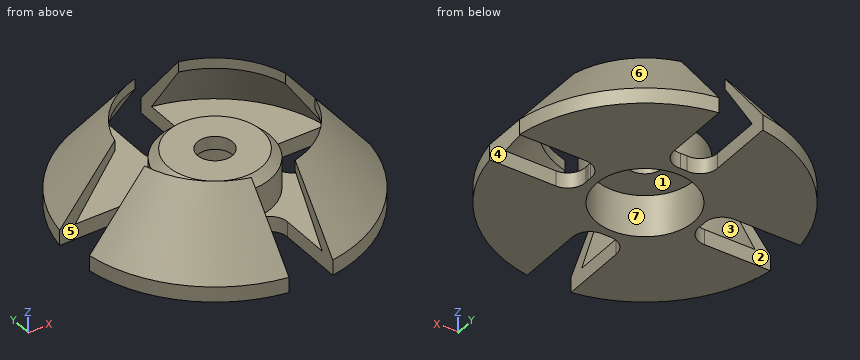
```python
from build123d import *

# Parameters (mm, degrees)
F0_R      = 32.5
F0_R_2    = 12.65
F0_R_3    = 11.15
F1_DEPTH  = 3.5
F2_DEPTH  = 9
F3_R      = 11.15
F3_R_2    = 4
F4_DEPTH  = 3
F5_SIZE   = 2
F10_DEPTH = 25
F11_DEPTH = 15.2
F12_R     = 4


with BuildPart() as f1:
    # F0 (on Top) → F1 (new body)
    with BuildSketch(Plane.XY):
        Circle(F0_R)
        Circle(F0_R_2, mode=Mode.SUBTRACT)
        Circle(F0_R_2)
        Circle(F0_R_3, mode=Mode.SUBTRACT)
    extrude(amount=-F1_DEPTH)

    # F0 (on Top) → F2 (join)
    with BuildSketch(Plane.XY):
        Circle(F0_R_2)
        Circle(F0_R_3, mode=Mode.SUBTRACT)
    extrude(amount=F2_DEPTH)

    # F3 (on face) → F4 (join)
    with BuildSketch(Plane.XY.offset(9)):
        Circle(F3_R)
        Circle(F3_R_2, mode=Mode.SUBTRACT)
    extrude(amount=-F4_DEPTH)

    # F5
    f5_edges = [f1.edges().sort_by_distance(p)[0] for p in [
        (-12.65, 0, 9),
    ]]
    chamfer(f5_edges, length=F5_SIZE)

    # F6 (on Front) → F7 (revolve)
    with BuildSketch(Plane.XZ):
        Polygon((-20.1347596889, 15.719441213), (-32.5, 0), (-29, 0), (-20.1347596889, 13.319441213), align=None)
    revolve(axis=Axis((0, 0, 0), (0, 0, -1)))

    # F9 (on offset) → F10 (cut)
    with BuildSketch(Plane.XY.offset(9)):
        with BuildLine():
            Line((5, 35), (-5, 35))
            Line((-5, 35), (-5, 12))
            ThreePointArc((-5, 12), (0, 13), (5, 12))
            Line((5, 12), (5, 35))
        make_face()
        with BuildLine():
            Line((35, 5), (12, 5))
            ThreePointArc((12, 5), (12.747548784, 2.5495097568), (13, 0))
            ThreePointArc((13, 0), (12.747548784, -2.5495097568), (12, -5))
            Line((12, -5), (35, -5))
            Line((35, -5), (35, 5))
        make_face()
        with BuildLine():
            ThreePointArc((5, -12), (0, -13), (-5, -12))
            Line((-5, -12), (-5, -35))
            Line((-5, -35), (5, -35))
            Line((5, -35), (5, -12))
        make_face()
        with BuildLine():
            ThreePointArc((-12, -5), (-13, 0), (-12, 5))
            Line((-12, 5), (-35, 5))
            Line((-35, 5), (-35, -5))
            Line((-35, -5), (-12, -5))
        make_face()
    extrude(amount=F10_DEPTH, mode=Mode.SUBTRACT)

    # F9 (on offset) → F11 (cut)
    with BuildSketch(Plane.XY.offset(9)):
        with BuildLine():
            ThreePointArc((5, -12), (0, -13), (-5, -12))
            Line((-5, -12), (-5, -35))
            Line((-5, -35), (5, -35))
            Line((5, -35), (5, -12))
        make_face()
        with BuildLine():
            Line((5, 35), (-5, 35))
            Line((-5, 35), (-5, 12))
            ThreePointArc((-5, 12), (0, 13), (5, 12))
            Line((5, 12), (5, 35))
        make_face()
        with BuildLine():
            ThreePointArc((-12, -5), (-13, 0), (-12, 5))
            Line((-12, 5), (-35, 5))
            Line((-35, 5), (-35, -5))
            Line((-35, -5), (-12, -5))
        make_face()
        with BuildLine():
            Line((35, 5), (12, 5))
            ThreePointArc((12, 5), (12.747548784, 2.5495097568), (13, 0))
            ThreePointArc((13, 0), (12.747548784, -2.5495097568), (12, -5))
            Line((12, -5), (35, -5))
            Line((35, -5), (35, 5))
        make_face()
    extrude(amount=-F11_DEPTH, mode=Mode.SUBTRACT)

    # F12
    f12_edges = [f1.edges().sort_by_distance(p)[0] for p in [
        (-12, 5, -1.75),
        (-12, -5, -1.75),
        (-5, 12, -1.75),
        (5, 12, -1.75),
        (-5, -12, -1.75),
        (5, -12, -1.75),
        (12, -5, -1.75),
        (12, 5, -1.75),
    ]]
    fillet(f12_edges, radius=F12_R)


solid = f1.part
```
Input: part model. Units: mm. Frame: model coordinates. Face numbers are marked on the shaded views. A direction names the side the tool comes from. Round coordinates to 2 decimals unless told otherwise and drop trailing zeros. Loops run counter-clockwise (first coordinate to the right, second up) from the corner with the lowest first, then second, coordinate; pieces in that order, holes last. Notation, with made-up numbers: M -27.5,-18.75 L 23.5,-18.75 A10 cw 23.5,-4.75 Z; hole C 42.5,-28 d6. An arc over 180 degrees is marked long. Answer in a Markdown table with one row per item. Add a question column.
1. Ray query, probe 1 along X at (y, z) = (7.5, 3); probe 2 along Y at (x, z) = (7.5, 1); probe 3 along Z at (x, y) = (6.5, 3.5). Return the intervals inside material, ascending.
2. Section B-B (z = 3). Output: boundary loops of the cut face in (x, y).
3. Set-up query: the marked faces 1, 2, 3 and 4. Return all of +Z, -Z, +X, -X, +Y, -Y with unobstructed straight access to the full face (end or side cutting, diameter ignored); none if empty.
4. Contact query for flat-ended pins moving along their axis: pin 1 (1 mm diameter, centred on x = -19.5, z = 8.5, fed in from -Y); pin 2 (4.5 mm diameter, centred on y = 21.5, z = 6.5, fed in from -X); pin 3 (5 mm diameter, centred on y = 10.5, z = 1.5, fed in from +X). Output: stop coordinate, or through.
5. Section C-C (z = 11). Output: boundary loops of the cut face in (x, y), and give its area (3 significant figures).
6. Mould query, pull axis X, two halves, no side actions, for the marked faces 5, 6 and 7. Classes: released by +X, released by -X, zero draft, split by the parting line, or undercut.
7. Section A-A (x = 0). Output: boundary loops of the cut face in (y, z), and give its area (4 significant figures).
Values follow:
| question | item | result |
|---|---|---|
| 1 | probe 1 | -29.19 to -25.94, -10.19 to -8.25, 8.25 to 10.19, 25.94 to 29.19 |
| 1 | probe 2 | -30.81 to -27.32, -10.19 to -8.25, 8.25 to 10.19, 27.32 to 30.81 |
| 1 | probe 3 | 6 to 9 |
| 2 | outline | M -29.72,-5 A30.14 ccw -5,-29.72 L -5,-26.54 A27 cw -26.54,-5 Z; M -29.72,5 L -26.54,5 A27 cw -5,26.54 L -5,29.72 A30.14 ccw Z; C 0,0 d25.3; M 5,-29.72 A30.14 ccw 29.72,-5 L 26.54,-5 A27 cw 5,-26.54 Z; M 5,26.54 A27 cw 26.54,5 L 29.72,5 A30.14 ccw 5,29.72 Z; hole C 0,0 d22.3 |
| 3 | face 1 | -Z |
| 3 | face 2 | +Z, -Z, -X |
| 3 | face 3 | none |
| 3 | face 4 | +Z, -Z, +X |
| 4 | pin 1 | y = -17.73 |
| 4 | pin 2 | x = -20.59 |
| 4 | pin 3 | x = 31.37 |
| 5 | outline | M -23.32,-5 A23.85 ccw -5,-23.32 L -5,-21.09 A21.68 cw -21.09,-5 Z; M -23.32,5 L -21.09,5 A21.68 cw -5,21.09 L -5,23.32 A23.85 ccw Z; M 5,-23.32 A23.85 ccw 23.32,-5 L 21.09,-5 A21.68 cw 5,-21.09 Z; M 5,21.09 A21.68 cw 21.09,5 L 23.32,5 A23.85 ccw 5,23.32 Z |
| 5 | area | 223 mm^2 |
| 6 | face 5 | zero draft |
| 6 | face 6 | released by +X |
| 6 | face 7 | undercut |
| 7 | outline | M -13,-3.5 L -11.15,-3.5 L -11.15,6 L -4,6 L -4,9 L -10.65,9 L -12.65,7 L -12.65,0 L -13,0 Z; M 4,6 L 11.15,6 L 11.15,-3.5 L 13,-3.5 L 13,0 L 12.65,0 L 12.65,7 L 10.65,9 L 4,9 Z |
| 7 | area | 78.85 mm^2 |
